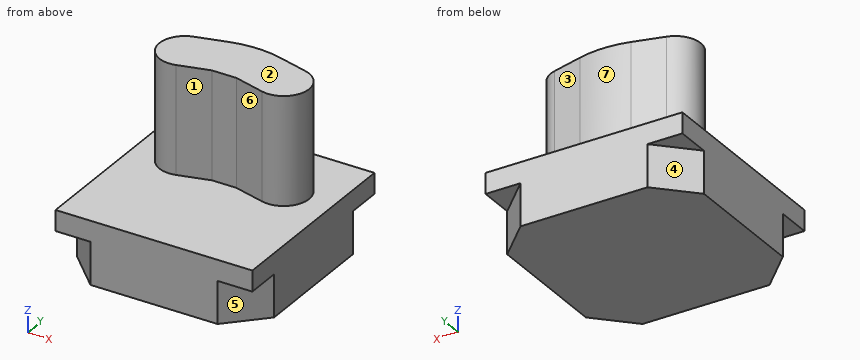
Autodesk Inventor part; units mm, degrees
ref_plane "YZ Plane" through (0, 0, 0) normal (1, 0, 0) x (0, 1, 0)
ref_plane "XZ Plane" through (0, 0, 0) normal (0, 1, 0) x (-1, 0, 0)
ref_plane "XY Plane" through (0, 0, 0) normal (0, 0, 1) x (1, 0, 0)
sketch "Sketch1" plane through (0, 0, 0) normal (0, 0, 1) x (1, 0, 0)
  line L0 (-310, 185.5) -> (310, 185.5)
  line L1 (310, 185.5) -> (310, -434.5)
  line L2 (310, -434.5) -> (-310, -434.5)
  line L3 (-310, -434.5) -> (-310, 185.5)
  point P0 (0, 0)
  point P1 (0, 185.5)
  dimension "d0" = 620
  dimension "d1" = 620
  dimension "d2" = 185.5
extrude "Extrusion1" add sketch "Sketch1" along normal mid plane 198
sketch "Sketch2" plane through (0, 0, -99) normal (0, 0, -1) x (-1, 0, 0)
  line L0 (-310, 185.5) -> (310, 185.5)
  line L1 (-310, 185.5) -> (-310, 75.5)
  line L2 (-310, -434.5) -> (-310, 185.5)
  line L3 (-310, 75.5) -> (-200, 185.5)
  line L4 (-310, 185.5) -> (-200, 185.5)
  line L5 (-310, -124.5) -> (0, -124.5)
  line L6 (0, -124.5) -> (0, 185.5)
  line L7 (-310, -434.5) -> (-310, -324.5)
  line L8 (-310, -434.5) -> (-200, -434.5)
  line L9 (-200, -434.5) -> (-310, -324.5)
  line L10 (310, -434.5) -> (200, -434.5)
  line L11 (310, -434.5) -> (310, -324.5)
  line L12 (310, -324.5) -> (200, -434.5)
  line L13 (310, 185.5) -> (310, 75.5)
  line L14 (310, 185.5) -> (200, 185.5)
  line L15 (200, 185.5) -> (310, 75.5)
  point P0 (0, 0)
  dimension "d5" = 110
  dimension "d6" = 110
  dimension "d9" = 360
extrude "Extrusion2" cut sketch "Sketch2" against normal blind 133 contours L0 L13 L15 | L9 L8 L2 | L0 L3 L1 | L10 L12 L11
sketch "Sketch3" plane through (0, 0, 99) normal (0, 0, 1) x (1, 0, 0)
  circle A0 centre (-155.8871, -26.656) radius 80 construction
  line L0 (-176.5926, 50.6181) -> (-80, 76.5)
  line L1 (-135.1815, -103.93) -> (-38.589, -78.0481)
  line L2 (-80, 76.5) -> (-38.589, -78.0481) construction
  line L3 (-80, 76.5) -> (80, 76.5) construction
  line L4 (80, 76.5) -> (38.589, -78.0481) construction
  line L5 (-38.589, -78.0481) -> (38.589, -78.0481)
  circle A1 centre (155.8871, -26.656) radius 80 construction
  line L6 (38.589, -78.0481) -> (135.1815, -103.93)
  line L7 (80, 76.5) -> (176.5926, 50.6181)
  arc A2 (-176.5926, 50.6181) -> (-135.1815, -103.93) centre (-155.8871, -26.656) ccw
  arc A3 (135.1815, -103.93) -> (176.5926, 50.6181) centre (155.8871, -26.656) ccw
  circle A4 centre (-155.8871, -26.656) radius 5.25
  circle A5 centre (155.8871, -26.656) radius 5.25
  line L8 (-106.5, 56.5) -> (-106.5, -56.5)
  line L9 (-106.5, -56.5) -> (106.5, -56.5)
  line L10 (106.5, -56.5) -> (106.5, 56.5)
  line L11 (106.5, 56.5) -> (-106.5, 56.5)
  arc A6 (80, 76.5) -> (-80, 76.5) centre (0, -228.172) ccw
  circle A7 centre (0, 71.664) radius 5.25
  line L12 (310, -434.5) -> (310, 185.5) construction
  line L13 (310, 185.5) -> (-310, 185.5) construction
  line L14 (0, 185.5) -> (0, 0) construction
  line L15 (0, 0) -> (310, 0) construction
  line L16 (310, 75.5) -> (310, -324.5) construction
  line L17 (0, -78.0481) -> (0, -56.5)
  point P0 (0, 76.5)
  point P1 (-106.5, 0)
  dimension "d32" = 160
  dimension "d33" = 100
  dimension "d34" = 100
  dimension "d35" = 160
  dimension "d36" = 160
  dimension "d37" = 160
  dimension "d38" = 75
  dimension "d39" = 75
  dimension "d40" = 160
  dimension "d41" = 100
  dimension "d42" = 100
  dimension "d43" = 10.5
  dimension "d44" = 10.5
  dimension "d45" = 113
  dimension "d46" = 213
  dimension "d47" = 20
  dimension "d48" = 315
  dimension "d49" = 10.5
  dimension "d50" = 15.164
  dimension "d51" = 185.5
extrude "Extrusion3" add sketch "Sketch3" along normal blind 339 contours L9 L8 L11 L10 | L0 A6 L7 A3 L6 L5 L1 A2 | A4 | A5 | A7
properties part number "Base" material "ABS Plastic"
The listing builds one solid part. Answer for the finished solid, in the listing's coordinates (mm). Face numbers are marked on the shaded views. A direction names the side the tool comes from. Round coordinates to 2 decimals unless told otherwise and drop trailing zeros. Loops run counter-clockwise (first coordinate to the right, second up) from the corner with the lowest first, then second, coordinate; pieces in that order, holes last.
Q1. Given pin 1 Ø1.5 at (x, y) = (244, -224) entering from +Z; pin 2 Ø3 at (x, z) = (76, 279.5) entering from +Y, each flat-ended and moving along its own axis, determine where each tip first touches the part or whether it passes through.
Q2. Section A-A, the plane y = -358 is taken. Determine the outline of the cut face in (x, z).
Q3. Section B-B, the plane z = 290 is taken. Determine the outline of the cut face in (x, y), then the cut area to 3 significant figures.
Q4. Which of the six approach directions +Z, -Z, +X, -X, +Y, -Y give full straight-line access (tool end or side, diameter ignored) to the marked faces 4, 5, 6 and 7?
Q5. Find the intervals of material crossed by line 1 (Z direction, x = 42.5, y = -251.5); line 2 (Y direction, x = 134, z = 241); line 3 (X direction, y = 9, z = 129.5), in increasing order.
Q6. Section C-C, the plane y = -232.5 is taken. Determine the outline of the cut face in (x, z).
Q7. For a pull along X with two mould halves and no side action, classify the marked faces 1, 2 and 3 as released by +X, released by -X, zero draft, split by the parting line, or undercut.
Completed:
1. pin 1: stops at z = 99
1. pin 2: stops at y = 77.89
2. outline: (-310, 34) - (-276.5, 34) - (-276.5, -99) - (276.5, -99) - (276.5, 34) - (310, 34) - (310, 99) - (-310, 99) - close
3. outline: (-176.59, 50.62) arc R80 ccw to (-135.18, -103.93) - (-38.59, -78.05) - (38.59, -78.05) - (135.18, -103.93) arc R80 ccw to (176.59, 50.62) - (80, 76.5) arc R315 ccw to (-80, 76.5) - close
3. area: 71,500 mm2
4. face 4: -Z, -X, +Y
4. face 5: -Z, +X, -Y
4. face 6: +Z, -Y
4. face 7: +Z, +Y
5. line 1: z = -99 to 99
5. line 2: y = -103.61 to 62.03
5. line 3: x = -227.5 to 227.5
6. outline: (-310, -99) - (310, -99) - (310, 99) - (-310, 99) - close
7. face 1: undercut
7. face 2: zero draft
7. face 3: released by +X
